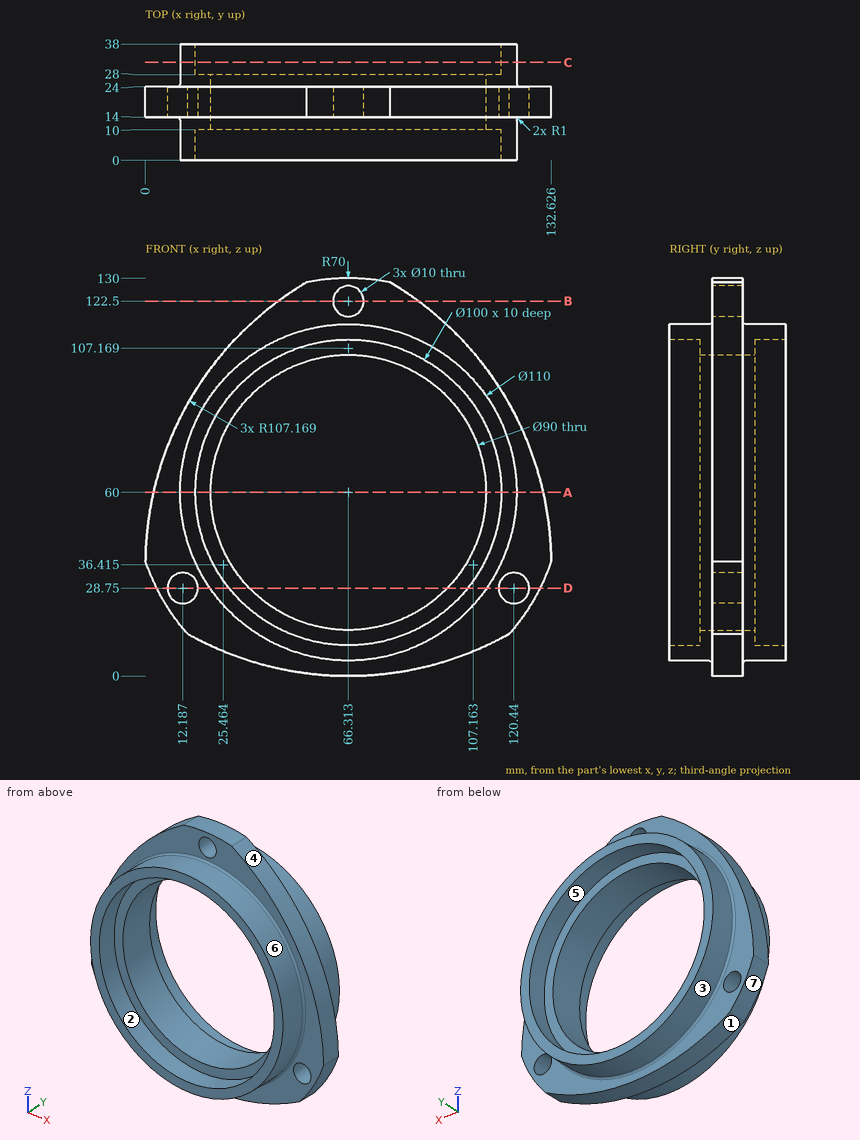
Print and shaded views of the part. All mm, measured from the part's lowest x, y and z. A direction names the side the tool comes from. Round coordinates to 2 decimals unless told otherwise and drop trailing zeros. Write each loop counter-clockwise with the first axis right and the second up, starting at its lowest first coordinate (ties: lowest second). Pieces come first, ordered by that corner, then holes. Notation, with made-up numbers: (38.5, 80.5) -> (66.5, 80.5) arc R7 ccw to (66.5, 90.5) -> close; hole circle Ø11 at (-14, -10). An arc over 180 degrees is marked (long way). Return JSON: item names as keys, results as strings. Group by question number.
Q1. Mould opens along Z. For the marked faces 4, 5, 6 and 7 say: pulls with the +Z half, pulls with the -Z half, needs draft (parallel to the pull), parting line crosses it, or undercut.
Q2. Saw through at D-D on z = 28.75. State how many separate pieces and enclosed holes the cut face has.
Q3. Saw through at A-A on z = 60. Write the cut outline in (x, y) (1 decimal).
Q4. Saw through at C-C on y = 32. Write the cut outline in (x, z).
Q5. Probe L1, parallel to X at y = 6, z = 60; L2, parallel to Y at x = 109, z = 20; L3, parallel to Z at x = 92, y = 28.5 (1 decimal). List the from-to ranges inside material, lowest first. Write a range as [from, to].
Q6. Pin check, flat tips, straight feed: pin 1 (1.5 mm diameter, centred on x = 100.5, y = 26, fed in from +Z); pin 2 (9 mm diameter, centred on x = 12.19, z = 28.75, fed in from -Y); pin 3 (4 mm diameter, centred on x = 45, y = 6.5, fed in from +Z); pin 4 (5 mm diameter, centred on x = 112, y = 14, fed in from -Z). Stop position of each tip, or through.
Q7. Saw through at B-B on z = 122.5. Write the cut outline in (x, y).
Q8. Which spindle directions (+Z, -Z, +X, -X, +Y, -Y) get a long thin tool onto all of the face, cutting with end or side? Do the marked faces 1, 2 and 3. Say none if no direction does.
Answer:
{
 "1": {"face 4": "pulls with the +Z half", "face 5": "undercut", "face 6": "parting line crosses it", "face 7": "pulls with the -Z half"},
 "2": {"separate pieces": "4", "enclosed holes": "0"},
 "3": {"outline": "(2.6, 14) -> (10.3, 14) arc R1 cw to (11.3, 13) -> (11.3, 0) -> (16.3, 0) -> (16.3, 10) -> (21.3, 10) -> (21.3, 28) -> (16.3, 28) -> (16.3, 38) -> (11.3, 38) -> (11.3, 25) arc R1 cw to (10.3, 24) -> (2.6, 24) -> close; (111.3, 10) -> (116.3, 10) -> (116.3, 0) -> (121.3, 0) -> (121.3, 13) arc R1 cw to (122.3, 14) -> (130, 14) -> (130, 24) -> (122.3, 24) arc R1 cw to (121.3, 25) -> (121.3, 38) -> (116.3, 38) -> (116.3, 28) -> (111.3, 28) -> close"},
 "4": {"outline": "circle Ø110 at (66.31, 60); hole circle Ø100 at (66.31, 60)"},
 "5": {"L1": "[11.31, 16.31], [116.31, 121.31]", "L2": "[14, 24]", "L3": "[11.4, 17.1], [102.9, 108.6]"},
 "6": {"pin 1": "z = 103.67", "pin 2": "through", "pin 3": "z = 111.5", "pin 4": "z = 9.09"},
 "7": {"outline": "(43.33, 14) -> (61.31, 14) -> (61.31, 24) -> (43.33, 24) -> close; (71.31, 14) -> (89.3, 14) -> (89.3, 24) -> (71.31, 24) -> close"},
 "8": {"face 1": "-Z, +Y, -Y", "face 2": "-Y", "face 3": "+Y"}
}
